from build123d import *

# Parameters (mm, degrees)
F0_W     = 50.8
F0_H     = 38.1
F1_DEPTH = 31.75
F3_DEPTH = 50.8
F4_W     = 25.4
F4_H     = 19.05
F5_DEPTH = 50.8


with BuildPart() as f1:
    # F0 (on Front) → F1 (new body)
    with BuildSketch(Plane.XZ):
        with Locations((-34.532589, 19.05)):
            Rectangle(F0_W, F0_H)
    extrude(amount=F1_DEPTH)

    # F2 (on face) → F3 (cut)
    with BuildSketch(Plane.YZ.offset(-9.132589)):
        with BuildLine():
            Line((-31.75, 38.1), (-31.75, 12.7))
            ThreePointArc((-31.75, 12.7), (-13.759905, 20.109905), (-6.35, 38.1))
            Line((-6.35, 38.1), (-31.75, 38.1))
        make_face()
    extrude(amount=-F3_DEPTH, mode=Mode.SUBTRACT)

    # F4 (on face) → F5 (cut)
    with BuildSketch(Plane(origin=(0, 0, 0), x_dir=(-1, 0, 0), z_dir=(0, 1, 0))):
        with Locations((34.532589, 28.575)):
            Rectangle(F4_W, F4_H)
    extrude(amount=-F5_DEPTH, mode=Mode.SUBTRACT)


solid = f1.part
Build history of the part. All positions in model axes, mm. A direction names the side the tool comes from. Coordinates: 2 decimals unless noted, no trailing zeros. Order: outer loops, then holes, each group sorted by start corner. A loop starts at its lowest first (then second) coordinate and runs counter-clockwise, first axis right, second up. Notation, with made-up numbers: (36.5, 26) - (65.5, 26) arc R14 ccw to (65.5, 46) - close; hole circle Ø3 at (0, 10.5). An arc over 180 degrees is marked (long way). Write each question's results on one line, items separated by ' | '. Start each with the question number.
Item 1: Tool access for faces 5 (the face through (-35, 0, 15)), 6 (the face through (-34, -7, 19.05)): list every direction of +Z, -Z, +X, -X, +Y, -Y with a clear straight run to the whole face (end or side of a thin tool).
Item 2: Band-saw the part on A-A on y = -2. Write the cut outline in (x, z).
Item 3: Band-saw the part on C-C on z = 35. Write the cut outline in (x, y), and give its area (3 significant figures).
Item 4: Band-saw the part on B-B on x = -17. Write the cut outline in (y, z), and give its area (3 significant figures).
Item 5: Mould opens along X. For faces 1 (the face through (-9.133, -12, 15)), 2 (the face through (-21.833, -4, 26)), 3 (the face through (-16, -3, 38.1)), 4 (the face through (-47.233, -4, 26)) say: released by +X, released by -X, zero draft, split by the parting line, or undercut.
Item 6: Band-saw the part on D-D on z = 29. Write the cut outline in (x, y), and give its area (3 significant figures).
Item 7: Wall check: probe 1 along X at (y, z) = (-7.5, 23.5); probe 2 along Z at (x, y) = (-34.5, -4); probe 3 along Z at (x, y) = (-19, -14). Give the ranges that are in metal, low to high. Write a range as [from, to].
Item 8: Flat gauge pins, fed straight in: pin 1 (1.5 mm diameter, centred on x = -51.5, z = 24, fed in from -Y); pin 2 (12 mm diameter, centred on x = -28.5, z = 30.5, fed in from +Y); pin 3 (3 mm diameter, centred on x = -34, y = -16, fed in from +Z); pin 4 (2 mm diameter, centred on x = -39, y = -28.5, fed in from +Z). Where does each tip first touch, or does it go through?
Numbers:
1) face 5: +Z, -Z, +X, -X, +Y | face 6: +Z, +Y, -Y
2) outline: (-59.93, 0) - (-9.13, 0) - (-9.13, 38.1) - (-21.83, 38.1) - (-21.83, 19.05) - (-47.23, 19.05) - (-47.23, 38.1) - (-59.93, 38.1) - close
3) outline: (-59.93, -6.53) - (-47.23, -6.53) - (-47.23, 0) - (-59.93, 0) - close; (-21.83, -6.53) - (-9.13, -6.53) - (-9.13, 0) - (-21.83, 0) - close | area: 166 mm^2
4) outline: (-31.75, 0) - (0, 0) - (0, 38.1) - (-6.35, 38.1) arc R25.3 cw to (-31.75, 12.7) - close | area: 702 mm^2
5) face 1: released by +X | face 2: undercut | face 3: zero draft | face 4: undercut
6) outline: (-59.93, -8) - (-47.23, -8) - (-47.23, 0) - (-59.93, 0) - close; (-21.83, -8) - (-9.13, -8) - (-9.13, 0) - (-21.83, 0) - close | area: 203 mm^2
7) probe 1: [-59.93, -47.23], [-21.83, -9.13] | probe 2: [0, 19.05] | probe 3: [0, 19.87]
8) pin 1: y = -11.09 | pin 2: through | pin 3: z = 19.05 | pin 4: z = 13.04
